```python
from build123d import *

# Parameters (mm, degrees)
SKETCH1_W               = 35
SKETCH1_H               = 30
BOSS_EXTRUDE1_DEPTH     = 28
SKETCH2_R               = 1.5
CUT_EXTRUDE1_DEPTH      = 10
SKETCH5_R               = 11.5
CUT_EXTRUDE4_DEPTH      = 3
CUT_EXTRUDE5_DEPTH      = 35.003676272
CUT_EXTRUDE5_DEPTH_BACK = 35.003676272
SKETCH6_R               = 4.5


with BuildPart() as part:
    # Sketch1 → Boss-Extrude1 (new body)
    with BuildSketch(Plane(origin=(0, 0, 0), x_dir=(1, 0, 0), z_dir=(0, 1, 0))):
        Rectangle(SKETCH1_W, SKETCH1_H)
    extrude(amount=BOSS_EXTRUDE1_DEPTH)

    # Sketch2 → Cut-Extrude1 (cut)
    with BuildSketch(Plane.XY.offset(15)):
        with Locations((-12.5, 23)):
            Circle(SKETCH2_R)
        with Locations((12.5, 23)):
            Circle(SKETCH2_R)
        with Locations((12.5, 5)):
            Circle(SKETCH2_R)
        with Locations((-12.5, 5)):
            Circle(SKETCH2_R)
    extrude(amount=-CUT_EXTRUDE1_DEPTH, mode=Mode.SUBTRACT)

    # Sketch5 → Cut-Extrude4 (cut)
    with BuildSketch(Plane.XZ):
        with Locations(Location((0, 0, 0), (0, 0, 270))):
            Circle(SKETCH5_R)
    extrude(amount=-CUT_EXTRUDE4_DEPTH, mode=Mode.SUBTRACT)

    # Sketch6 → Cut-Extrude5 (cut, two sides: drawn at the far end of the back side and taken through both)
    with BuildSketch(Plane(origin=(0, 3, 0), x_dir=(-1, 0, 0), z_dir=(0, -1, 0)).offset(-CUT_EXTRUDE5_DEPTH_BACK)):
        with Locations(Location((0, 0, 0), (0, 0, 90))):
            Circle(SKETCH6_R)
    extrude(amount=CUT_EXTRUDE5_DEPTH + CUT_EXTRUDE5_DEPTH_BACK, mode=Mode.SUBTRACT)


solid = part.part
```
CAD build for the part. Positions are in the model's coordinates, mm. A direction names the side the tool comes from. Round coordinates to 2 decimals unless told otherwise and drop trailing zeros. Loops run counter-clockwise (first coordinate to the right, second up) from the corner with the lowest first, then second, coordinate; pieces in that order, holes last. Notation, with made-up numbers: M 82,76 L 133,76 A20 cw 133,82 Z; hole C 87.5,86.5 d4. An arc over 180 degrees is marked long. Return JSON: item names as keys, results as strings. Group by question number.
(1) Saw through at B-B, the plane z = 0. List the corners of the cut face in (x, y).
(2) Saw through at D-D, the plane z = -6.75. List the corners of the cut face in (x, y).
(3) Mould opens along Z. For faces 4 (the flat face through (0, 3, -5)), 5 (the flat face through (17.5, 14, 0)), 6 (the flat face through (0, 14, -15)) say: +Z half, -Z half, draft (parallel to the pull), parting line (faces both ways), or undercut.
(4) Saw through at A-A, the plane y = 5. List the corners of the cut face in (x, z).
(5) Drop flat-ended pins along their axis: P1, Ø6, axis at x = -6, z = 3, coming from the -Y side; P2, Ø0.9, axis at x = 12, y = 5.5, coming from the +Z side. Give the stop position or say it passes through.
(6) Saw through at C-C, the plane x = -12.5. List the corners of the cut face in (y, z), and give its area (3 significant figures).
(7) Wall check: probe 1 along Y at (x, z) = (12.5, 8); probe 2 along X at (y, z) = (11.5, 0); probe 3 along Y at (x, z) = (-13, 13.75). Give the ranges that are in metal, low to high. Write a range as [from, to].
(8) Tool access for faces 1 (the cylindrical face through (9.7, 1.48, -6.18)), 2 (the flat face through (-12, 0, 0)), 3 (the cylindrical face through (-14, 5, 10)): list every direction of +Z, -Z, +X, -X, +Y, -Y with a clear straight run to the whole face (end or side of a thin tool).
Answer list:
{
 "1": {"outline": "M -17.5,0 L -11.5,0 L -11.5,3 L -4.5,3 L -4.5,28 L -17.5,28 Z; M 4.5,3 L 11.5,3 L 11.5,0 L 17.5,0 L 17.5,28 L 4.5,28 Z"},
 "2": {"outline": "M -17.5,0 L -9.31,0 L -9.31,3 L 9.31,3 L 9.31,0 L 17.5,0 L 17.5,28 L -17.5,28 Z"},
 "3": {"face 4": "undercut", "face 5": "draft", "face 6": "-Z half"},
 "4": {"outline": "M -17.5,-15 L 17.5,-15 L 17.5,15 L 14,15 L 14,5 L 11,5 L 11,15 L -11,15 L -11,5 L -14,5 L -14,15 L -17.5,15 Z; hole C 0,0 d9"},
 "5": {"P1": "y = 3", "P2": "z = 5"},
 "6": {"outline": "M 0,-15 L 28,-15 L 28,15 L 24.5,15 L 24.5,5 L 21.5,5 L 21.5,15 L 6.5,15 L 6.5,5 L 3.5,5 L 3.5,15 L 0,15 Z", "area": "780 mm2"},
 "7": {"probe 1": "[0, 3.5], [6.5, 21.5], [24.5, 28]", "probe 2": "[-17.5, -4.5], [4.5, 17.5]", "probe 3": "[0, 3.59], [6.41, 21.59], [24.41, 28]"},
 "8": {"face 1": "-Y", "face 2": "+Z, -Z, +X, -X, -Y", "face 3": "+Z"}
}
